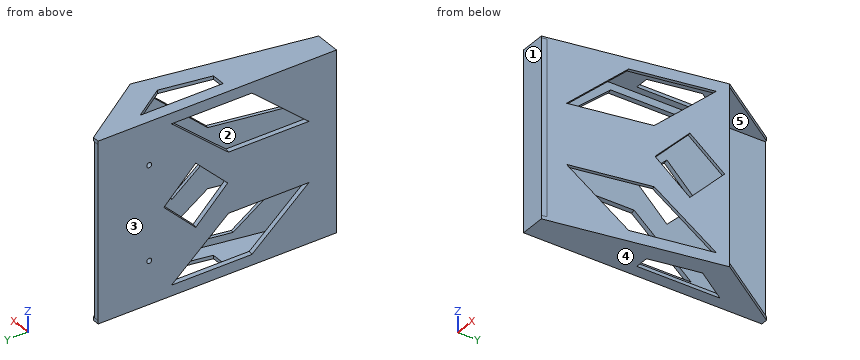
from build123d import *

# Parameters (mm, degrees)
BOSS_EXTRU_1_DEPTH         = 2
BOSS_EXTRU_2_DEPTH         = 102
R_P_TITION_LIN_AIRE1_COUNT = 2
R_P_TITION_LIN_AIRE1_PITCH = 103
ESQUISSE5_W                = 2.97567345
ESQUISSE5_H                = 101
BOSS_EXTRU_3_DEPTH         = 137
ESQUISSE6_W                = 2
ESQUISSE6_H                = 101
ESQUISSE9_R                = 1.462141601
ENL_V_MAT_EXTRU_8_DEPTH    = 10
ENL_V_MAT_EXTRU_10_DEPTH   = 178.957906594
ENL_V_MAT_EXTRU_11_DEPTH   = 178.957906594
ENL_V_MAT_EXTRU_12_DEPTH   = 178.97245401


with BuildPart() as part:
    # Esquisse2 → Boss.-Extru.1 (new body)
    with BuildSketch(Plane.XY):
        Polygon((0, 0), (0, 140), (3.942801894, 140), (32.364817767, 98.480775301), (15, 0), align=None)
    boss_extru_1 = extrude(amount=BOSS_EXTRU_1_DEPTH)

    # Esquisse4 → Boss.-Extru.2 (add)
    with BuildSketch(Plane.XY.offset(2)):
        Polygon((0, 0), (0, 3.006117571), (15.530059635, 3.006117571), (15, 0), align=None)
    extrude(amount=BOSS_EXTRU_2_DEPTH)

    # Répétition linéaire1: Boss.-Extru.1 ×2
    with Locations(*[(0, 0, i * R_P_TITION_LIN_AIRE1_PITCH) for i in range(1, R_P_TITION_LIN_AIRE1_COUNT)]):
        add(boss_extru_1)

    # Esquisse5 → Boss.-Extru.3 (add)
    with BuildSketch(Plane(origin=(0, 3.006117571, 0), x_dir=(1, 0, 0), z_dir=(0, 1, 0))):
        with Locations((1.487836725, -52.5)):
            Rectangle(ESQUISSE5_W, ESQUISSE5_H)
    extrude(amount=BOSS_EXTRU_3_DEPTH)

    # Balayage1: sweep along a curve in space
    with BuildLine() as balayage1_path:
        Line((15.530059635, 3.006117571, 103), (32.364817767, 98.480775301, 103))
    # Esquisse6 → Balayage1 (sweep)
    with BuildSketch(Plane(origin=(0, 3.006117571, 0), x_dir=(1, 0, 0), z_dir=(0, 1, 0))):
        with Locations((14.530059635, -52.5)):
            Rectangle(ESQUISSE6_W, ESQUISSE6_H)
    sweep(path=balayage1_path.line)

    # Esquisse9 → Enlèv. mat.-Extru.8 (cut)
    with BuildSketch(Plane(origin=(2.97567345, 0, 0), x_dir=(0, 0, -1), z_dir=(1, 0, 0))):
        with Locations((-80, 110)):
            Circle(ESQUISSE9_R)
    enl_v_mat_extru_8 = extrude(amount=-ENL_V_MAT_EXTRU_8_DEPTH, mode=Mode.SUBTRACT)

    # Symétrie3: Enlèv. mat.-Extru.8 across plane
    add(enl_v_mat_extru_8.mirror(Plane.XY.offset(52.5)), mode=Mode.SUBTRACT)

    # Esquisse11 → Enlèv. mat.-Extru.10 (cut, through all)
    with BuildSketch(Plane(origin=(14.547694656, -2.565151075, 0), x_dir=(0, 0, -1), z_dir=(0.9848077530122089, -0.17364817766692642, 0))):
        Polygon((-6.160430803, 48.968309083), (-6.160430803, 95.489627834), (-34.939480046, 62.478304571), (-34.939480046, 15.95698582), align=None)
    enl_v_mat_extru_10 = extrude(amount=-ENL_V_MAT_EXTRU_10_DEPTH, mode=Mode.SUBTRACT)

    # Symétrie4: Enlèv. mat.-Extru.10 across plane
    add(enl_v_mat_extru_10.mirror(Plane.XY.offset(52.5)), mode=Mode.SUBTRACT)

    # Esquisse13 → Enlèv. mat.-Extru.11 (cut, through all)
    with BuildSketch(Plane(origin=(14.547694656, -2.565151075, 0), x_dir=(0, 0, -1), z_dir=(0.9848077530122089, -0.17364817766692642, 0))):
        Polygon((-70.968675793, 81.423632051), (-52.5, 62.954956258), (-34.031324207, 81.423632051), (-52.5, 99.892307844), align=None)
    extrude(amount=-ENL_V_MAT_EXTRU_11_DEPTH, mode=Mode.SUBTRACT)

    # Esquisse14 → Enlèv. mat.-Extru.12 (cut, through all)
    with BuildSketch(Plane(origin=(0, 0, 0), x_dir=(-1, 0, 0), z_dir=(0, 0, -1))):
        Polygon((-7.076060975, 110.418465172), (-7.076060975, 61.600550279), (-15.271885521, 61.600550279), (-20.438019848, 90.899153967), align=None)
    extrude(amount=-ENL_V_MAT_EXTRU_12_DEPTH, mode=Mode.SUBTRACT)


solid = part.part
Geometry: final body of the model. Coordinates: model frame, mm. Face numbers are marked on the shaded views. A direction names the side the tool comes from. Coordinates: 2 decimals unless noted, no trailing zeros. Loops run counter-clockwise (first coordinate to the right, second up) from the corner with the lowest first, then second, coordinate; pieces in that order, holes last. Notation, with made-up numbers: (40.25, 79) - (64.25, 79) arc R21 ccw to (64.25, 93) - close; hole circle Ø7 at (28.5, 30). An arc over 180 degrees is marked (long way). Put each result on its own line as item: value. Start each with the question number.
Q1. Pull-direction query (X, two-part tool) for the marked faces 3, 4 and 5; classes: released by +X, released by -X, zero draft, split by the parting line, or undercut.
Q2. Cut plane C-C, the plane z = 58.5. Return loops of the section in (x, y).
Q3. Cut plane B-B, the plane z = 80. Return loops of the section in (x, y).
Q4. Line query: line 1 (Z direction, x = 1.8, y = 110); line 2 (Y direction, x = 1, z = 80); line 3 (Z direction, x = 16, y = 113.5). Output: solid intervals per line, ascending.
Q5. Set-up query: the marked faces 1 and 2. Return all of +Z, -Z, +X, -X, +Y, -Y with unobstructed straight access to the full face (end or side cutting, diameter ignored); none if empty.
Q6. Cut plane A-A, the plane y = 25.5. Return loops of the section in (x, z).
Q7. Cut plane D-D, the plane y = 67. Give the number of separate pieces and of enclosed holes in the cut face, and give its area (3 significant figures).
Q8. Pin query (flat end, axial travel): pin 1 Ø4 at (x, z) = (28.5, 86.5) entering from -Y; pin 2 Ø0.6 at (x, z) = (2.5, 0.5) entering from +Y; pin 3 Ø0.6 at (y, z) = (88.5, 0.5) entering from +X. Return the tip coordinate at first contact, or that it passes through.
Filled sheet:
1. face 3: released by -X
1. face 4: zero draft
1. face 5: undercut
2. outline: (0, 0) - (15, 0) - (26.52, 65.34) - (24.58, 65.68) - (13.53, 3.01) - (2.98, 3.01) - (2.98, 69.49) - (0, 70.02) - close; (0, 95.34) - (2.98, 94.82) - (2.98, 140.01) - (0, 140.01) - close; (28.91, 90.24) - (30.85, 89.9) - (32.36, 98.48) - (30.36, 98.48) - close
3. outline: (0, 0) - (15, 0) - (19.3, 24.38) - (17.36, 24.72) - (13.53, 3.01) - (2.98, 3.01) - (2.98, 27.26) - (0, 27.78) - close; (0, 75.02) - (2.98, 74.49) - (2.98, 108.54) - (0, 108.54) - close; (0, 111.46) - (2.98, 111.46) - (2.98, 140.01) - (0, 140.01) - close; (25.44, 70.53) - (27.38, 70.19) - (32.36, 98.48) - (30.36, 98.48) - close
4. line 1: 0 to 23.54, 26.46 to 78.54, 81.46 to 105
4. line 2: 0 to 27.6, 74.84 to 108.54, 111.46 to 140.01
4. line 3: 0 to 2, 103 to 105
5. face 1: +Z, -Z, +X, -X, -Y
5. face 2: +Y
6. outline: (0, 0) - (19.5, 0) - (19.5, 24.01) - (17.5, 24.31) - (17.5, 2) - (2.98, 2) - (2.98, 26.51) - (0, 26.96) - close; (0, 34.94) - (2.98, 34.94) - (2.98, 70.06) - (0, 70.06) - close; (0, 78.04) - (2.98, 78.49) - (2.98, 103) - (17.5, 103) - (17.5, 80.69) - (19.5, 80.99) - (19.5, 105) - (0, 105) - close; (17.5, 34.94) - (19.5, 34.94) - (19.5, 70.06) - (17.5, 70.06) - close
7. separate pieces: 8
7. enclosed holes: 0
7. area: 285 mm²
8. pin 1: y = 75.29
8. pin 2: y = 140
8. pin 3: x = 30.66
